```python
from build123d import *

# Parameters (mm, degrees)
F1_DEPTH  = 15
F2_R      = 14
F3_DEPTH  = 4
F4_R      = 2.1
F5_DEPTH  = 1.5
F7_R      = 0.5588
F8_DEPTH  = 12.7
F13_DEPTH = 3


with BuildPart() as f1:
    # F0 (on Top) → F1 (new body)
    with BuildSketch(Plane.XY):
        with BuildLine():
            Line((7.3, -25), (7.3, -19.946129))
            ThreePointArc((7.3, -19.946129), (0, 6), (-7.3, -19.946129))
            Line((-7.3, -19.946129), (-7.3, -25))
            Line((-7.3, -25), (7.3, -25))
        make_face()
    extrude(amount=-F1_DEPTH)

    # F2 (on face) → F3 (join)
    with BuildSketch(Plane(origin=(0, 0, -15), x_dir=(1, 0, 0), z_dir=(0, 0, -1))):
        with Locations((0, 8)):
            Circle(F2_R)
    extrude(amount=F3_DEPTH)

    # F4 (on Top) → F5 (join)
    with BuildSketch(Plane.XY):
        with BuildLine():
            ThreePointArc((-17.823718, -4.5), (-21.323718, -8), (-17.823718, -11.5))
            Line((-17.823718, -11.5), (17.823718, -11.5))
            ThreePointArc((17.823718, -11.5), (21.323718, -8), (17.823718, -4.5))
            Line((17.823718, -4.5), (-17.823718, -4.5))
        make_face()
        with Locations((-17.823718, -8)):
            Circle(F4_R, mode=Mode.SUBTRACT)
        with Locations((17.823718, -8)):
            Circle(F4_R, mode=Mode.SUBTRACT)
    extrude(amount=-F5_DEPTH)

    # F7 (on face) → F8 (join)
    with BuildSketch(Plane.XZ.offset(25)):
        with Locations((-2.8448, -5)):
            Circle(F7_R)
        with Locations((-1.4224, -5)):
            Circle(F7_R)
        with Locations((0, -5)):
            Circle(F7_R)
        with Locations((1.4224, -5)):
            Circle(F7_R)
        with Locations((2.8448, -5)):
            Circle(F7_R)
    extrude(amount=F8_DEPTH)

    # F9 (on Right) → F10 (revolve)
    with BuildSketch(Plane.YZ):
        Polygon((0, 7.5), (0, 0), (4.5, 0), (4.5, 1.5), (2.5, 1.5), (2.5, 7.5), align=None)
    revolve(axis=Axis((0, 0, 3.75), (0, 0, 1)))

    # F12 (on offset) → F13 (join, through all)
    with BuildSketch(Plane.XY.offset(10.5)):
        with BuildLine():
            Line((2, 1.5), (-2, 1.5))
            ThreePointArc((-2, 1.5), (-2.5, 0), (-2, -1.5))
            Line((-2, -1.5), (2, -1.5))
            ThreePointArc((2, -1.5), (2.5, 0), (2, 1.5))
        make_face()
    extrude(amount=-F13_DEPTH)


solid = f1.part
```
Check sheet for the modelled part. Datum: model origin and axes. Units: mm. A direction names the side the tool comes from. Coordinates: 2 decimals unless noted, no trailing zeros. Write each loop counter-clockwise with the first axis right and the second up, starting at its lowest first coordinate (ties: lowest second). Pieces come first, ordered by that corner, then holes. Notation, with made-up numbers: M -36.5,11 L -12.5,11 A6 cw -12.5,21 Z; hole C -14,51.5 d4. An arc over 180 degrees is marked long. Write item = value, one per line. Start each with the question number.
1. Sectioned sample at D-D (x = 0). Record the cut outline in (y, z), then the cut area to 3 significant figures.
2. Mould release check, pull along X, two halves, no side actions. Record for faces 1 (the flat face through (1.4, -37.7, -5)), 2 (the cylindrical face through (21.323, -8.077, -0.74)), 3 (the cylindrical face through (-18.1, -5.92, -0.74)): pulls with the +X half, pulls with the -X half, needs draft (parallel to the pull), parting line crosses it, or undercut.
3. Go/stop test with flat-tipped pins: pin 1 (0.8 mm diameter, centred on x = -15, z = -1, fed in from +Y); pin 2 (0.9 mm diameter, centred on x = -0.5, z = 9, fed in from -Y); pin 3 (1.1 mm diameter, centred on x = 0.5, y = 2, fed in from +Z); pin 4 (1.5 mm diameter, centred on y = -0.5, z = -2.5, fed in from +X). Record where each tip stops, or that it passes through.
4. Sectioned sample at B-B (z = -5). Record the cut outline in (x, y), then the cut area to 3 significant figures.
5. Sectioned sample at A-A (y = -8). Record the cut outline in (x, z).
6. Thickness scan on probe 1 along Y at (x, z) = (-15, -1.25); probe 2 along Z at (x, y) = (-1, -17); probe 3 along Y at (x, z) = (-7, -8.75). Record the ranges inside material, lowest first.
7. Tool access check on faces 4 (the cylindrical face through (-3.403, -31.261, -4.975)), 5 (the flat face through (7.3, -23, -7)), 6 (the flat face through (0, 1.5, 9)). Record the directions out of +Z, -Z, +X, -X, +Y, -Y that give a thin tool (end or side, any length) a straight path to the whole face; none if there is none.
8. Sectioned sample at C-C (x = -17). Record the cut outline in (y, z).
The answers:
q1.outline = M -37.7,-5.56 L -25,-5.56 L -25,-15 L -22,-15 L -22,-19 L 6,-19 L 6,0 L 4.5,0 L 4.5,1.5 L 2.5,1.5 L 2.5,7.5 L 1.5,7.5 L 1.5,10.5 L -1.5,10.5 L -1.5,7.5 L -2.5,7.5 L -2.5,1.5 L -4.5,1.5 L -4.5,0 L -25,0 L -25,-4.44 L -37.7,-4.44 Z
q1.area = 644 mm²
q2.face_1 = needs draft
q2.face_2 = pulls with the +X half
q2.face_3 = undercut
q3.pin_1 = -4.5
q3.pin_2 = -1.5
q3.pin_3 = 10.5
q3.pin_4 = 12.27
q4.outline = M -7.3,-25 L -3.4,-25 L -3.4,-37.7 L -2.29,-37.7 L -2.29,-25 L -1.98,-25 L -1.98,-37.7 L -0.86,-37.7 L -0.86,-25 L -0.56,-25 L -0.56,-37.7 L 0.56,-37.7 L 0.56,-25 L 0.86,-25 L 0.86,-37.7 L 1.98,-37.7 L 1.98,-25 L 2.29,-25 L 2.29,-37.7 L 3.4,-37.7 L 3.4,-25 L 7.3,-25 L 7.3,-19.95 A14 ccw long -7.3,-19.95 Z
q4.area = 740 mm²
q5.outline = M -21.32,-1.5 L -19.92,-1.5 L -19.92,0 L -21.32,0 Z; M -15.72,-1.5 L -14,-1.5 L -14,-19 L 14,-19 L 14,-1.5 L 15.72,-1.5 L 15.72,0 L -15.72,0 Z; M 19.92,-1.5 L 21.32,-1.5 L 21.32,0 L 19.92,0 Z
q6.probe_1 = -11.5 to -4.5
q6.probe_2 = -19 to 0
q6.probe_3 = -25 to 4.12
q7.face_4 = -Y
q7.face_5 = +Z, -Z, +X, -Y
q7.face_6 = +Z, +X, -X, +Y
q8.outline = M -11.5,-1.5 L -9.93,-1.5 L -9.93,0 L -11.5,0 Z; M -6.07,-1.5 L -4.5,-1.5 L -4.5,0 L -6.07,0 Z
